Autodesk Inventor part; units mm, degrees
ref_plane "YZ Plane" through (0, 0, 0) normal (1, 0, 0) x (0, 1, 0)
ref_plane "XZ Plane" through (0, 0, 0) normal (0, 1, 0) x (-1, 0, 0)
ref_plane "XY Plane" through (0, 0, 0) normal (0, 0, 1) x (1, 0, 0)
sketch "Sketch1" plane through (0, 0, 0) normal (0, 0, 1) x (1, 0, 0)
  line L0 (0, 0) -> (50, 0)
  line L1 (50, 0) -> (50, -25)
  line L2 (50, -25) -> (0, -25)
  line L3 (0, -25) -> (0, 0)
  line L4 (50, 0) -> (60, -12.5)
  line L5 (60, -12.5) -> (50, -25)
  line L6 (0, -25) -> (-10, -12.5)
  line L7 (-10, -12.5) -> (0, 0)
  circle A0 centre (55, -12.5) radius 1.15
  circle A1 centre (-5, -12.5) radius 1.15
  dimension "d0" = 50
  dimension "d1" = 25
  dimension "d18" = 12.5
  dimension "d19" = 10
  dimension "d20" = 10
  dimension "d21" = 2.3
  dimension "d22" = 2.3
  dimension "d23" = 5
  dimension "d24" = 5
extrude "Extrusion1" add sketch "Sketch1" along normal blind 2
sketch "Sketch4" plane through (0, 0, 2) normal (0, 0, 1) x (1, 0, 0)
  line L0 (2.15, -22.85) -> (47.85, -22.85)
  line L1 (47.85, -22.85) -> (47.85, -2.15)
  line L2 (47.85, -2.15) -> (2.15, -2.15)
  line L3 (2.15, -2.15) -> (2.15, -22.85)
  point P0 (0, 0)
  point P1 (2.15, -12.5)
  point P2 (50, -25)
  dimension "d25" = 20.7
  dimension "d26" = 2.15
  dimension "d27" = 45.7
  dimension "d28" = 2.15
extrude "Extrusion4" add sketch "Sketch4" along normal blind 2
sketch "Sketch5" plane through (0, 0, 4) normal (0, 0, 1) x (1, 0, 0)
  line L0 (0, -25) -> (50, -25)
  line L1 (31, -25) -> (19, -25)
  line L2 (19, -25) -> (19, -17)
  line L3 (19, -17) -> (31, -17)
  line L4 (31, -17) -> (31, -25)
  point P0 (0, 0)
  dimension "d31" = 19
  dimension "d32" = 12
  dimension "d33" = 8
extrude "Extrusion5" cut sketch "Sketch5" against normal through all
fillet "Fillet1" radius 4 2 edges at (-10, -12.5, 1) (60, -12.5, 1)
properties part number "UltrasonicSensorMountTest_backplate"
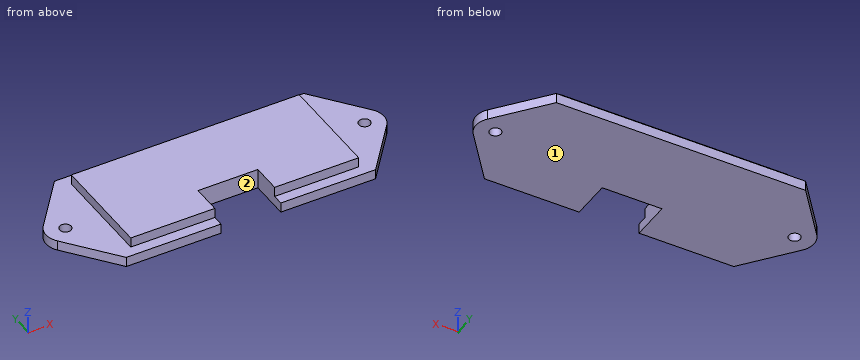
Model file for the job. Use its own axes, mm. Face numbers are marked on the shaded views. Round coordinates to 2 decimals unless told otherwise and drop trailing zeros. Order: outer loops, then holes, each group sorted by start corner. A loop starts at its lowest first (then second) coordinate and runs counter-clockwise, first axis right, second up.
(1) Pin check, flat tips, straight feed: pin 1 (2 mm diameter, centred on x = 38.5, z = 2.5, fed in from -Y); pin 2 (2 mm diameter, centred on x = 11.5, z = 3.5, fed in from -Y); pin 3 (3 mm diameter, centred on x = 55, y = -12.5, fed in from +Z); pin 4 (1.2 mm diameter, centred on y = -21, z = 3, fed in from -X). Stop position of each tip, or through.
(2) Band-saw the part on A-A (y = -18.5). List the corners of the cut face in (x, z), then the cut area to 3 significant figures.
(3) Drill centre lines: line 1 (Y direction, x = 31.5, z = 3.7); line 2 (Z direction, x = 0, y = -13.75); line 3 (X direction, y = -18.75, z = 0.25). Where is each one in solid material? Low to high.
(4) Band-saw the part on C-C (z = 0.8). List the corners of the cut face in (x, y).
(5) Band-saw the part on B-B (x = 55). List the corners of the cut face in (y, z).
(6) Band-saw the part on D-D (x = 27). List the corners of the cut face in (y, z), then the cut area to 3 significant figures.
(7) Pull direction X, two halves, no side cores. Call the marked faces 1 and 2: released by +X, released by -X, zero draft, split by the parting line, or undercut.
Verdict:
1. pin 1: stops at y = -25
1. pin 2: stops at y = -22.85
1. pin 3: stops at z = 2
1. pin 4: stops at x = 2.15
2. outline: (-5.2, 0) - (19, 0) - (19, 4) - (2.15, 4) - (2.15, 2) - (-5.2, 2) - close; (31, 0) - (55.2, 0) - (55.2, 2) - (47.85, 2) - (47.85, 4) - (31, 4) - close
2. area: 164 mm2
3. line 1: y = -22.85 to -2.15
3. line 2: z = 0 to 2
3. line 3: x = -5 to 19, 31 to 55
4. outline: (-8, -15) - (0, -25) - (19, -25) - (19, -17) - (31, -17) - (31, -25) - (50, -25) - (58, -15) arc R4 ccw to (58, -10) - (50, 0) - (0, 0) - (-8, -10) arc R4 ccw to start; hole circle Ø2.3 at (-5, -12.5); hole circle Ø2.3 at (55, -12.5)
5. outline: (-18.75, 0) - (-13.65, 0) - (-13.65, 2) - (-18.75, 2) - close; (-11.35, 0) - (-6.25, 0) - (-6.25, 2) - (-11.35, 2) - close
6. outline: (-17, 0) - (0, 0) - (0, 2) - (-2.15, 2) - (-2.15, 4) - (-17, 4) - close
6. area: 63.7 mm2
7. face 1: zero draft
7. face 2: undercut
